Source: CAD feature listing. Evaluate the final solid. Frame: model axes, mm. A direction names the side the tool comes from. Coordinates: 2 decimals unless noted, no trailing zeros. Order: outer loops, then holes, each group sorted by start corner. A loop starts at its lowest first (then second) coordinate and runs counter-clockwise, first axis right, second up. Notation, with made-up numbers: (28.5, -33) -> (42.5, -33) arc R24 cw to (42.5, -8) -> close; hole circle Ø4 at (85, 0). An arc over 180 degrees is marked (long way). Write item = value, one per line. Start each with the question number.
Item 1: Section query A-A (y = -108.25). Output: boundary loops of the cut face in (x, z).
Item 2: Set-up query: faces 1 (the flat face through (-10, 1, 2)), 2 (the flat face through (-10, 102, 6)), 3 (the flat face through (0.1, 104.6, 4)), 4 (the flat face through (3, -111, 8)), 5 (the flat face through (42, -62.5, 2)). Return all of +Z, -Z, +X, -X, +Y, -Y with unobstructed straight access to the full face (end or side cutting, diameter ignored); none if empty.
Item 3: Mould query, pull axis X, two halves, no side actions, for faces 6 (the flat face through (0, -101, 8.5)), 7 (the flat face through (-10, -101, 6)), 8 (the cylindrical face through (40.434, -40.958, 2.281)). Classes: released by +X, released by -X, zero draft, split by the parting line, or undercut.
Item 4: Section query C-C (x = 0). Count the separate pieces of the cut face and the enclosed holes in it, then the cut area to 3 significant figures.
Item 5: Section query B-B (y = 77.5). Output: boundary loops of the cut face in (x, z) (3 decimals).
Item 6: Ray query, line 1 along Y through (x, z) = (0, 6) (3 decimals); line 2 along Y through (x, z) = (68.5, 4); line 3 along Y through (x, z) = (-14, 2.5). Return the intervals inside material, ascending. Write a range as [from, to].
Item 7: Contact query for flat-ended pins moving along their axis: pin 1 (4 mm diameter, centred on x = 14, z = 4, fed in from -Y); pin 2 (4.5 mm diameter, centred on x = 14.375, y = -77.5, fed in from -Z); pin 3 (3.5 mm diameter, centred on x = -2, y = -107.5, fed in from +Z); pin 4 (17.5 mm diameter, centred on x = -4, y = -111, fed in from -Z). Output: stop coordinate, or through.
```python
from build123d import *
from OCP.BRepFilletAPI import BRepFilletAPI_MakeFillet

# Parameters (mm, degrees)
SKETCH_1_W                   = 20
SKETCH_1_H                   = 232
EXTRUDE_1_DEPTH              = 4.5
FILLET_4_R                   = 5
EXTRUDE_START                = 4
EXTRUDE_4_DEPTH              = 4
SKETCH_9_W                   = 319.021375536
SKETCH_9_H                   = 251.112704656
SKETCH_9_W_2                 = 165.944204682
SKETCH_9_H_2                 = 200
CUT_EXTRUDE_1_DEPTH          = 4
FILLET_5_R                   = 4
HOLE_WIZARD_M6_2_D           = 6.6
HOLE_WIZARD_M6_2_CBORE_D     = 12
HOLE_WIZARD_M6_2_CBORE_DEPTH = 0.5
SKETCH_12_W                  = 65
SKETCH_12_H                  = 125
SKETCH_12_R                  = 6.25
EXTRUDE_5_DEPTH              = 4.5
SKETCH_14_R                  = 22.5
EXTRUDE_6_DEPTH              = 4.5
FILLET_6_R1                  = 10
FILLET_6_R2                  = 22.5
SKETCH_13_R                  = 6.25
CUT_EXTRUDE_2_DEPTH          = 139.39526726
HOLE_WIZARD_M6_1_D           = 5
SKETCH_17_W                  = 35
SKETCH_17_H                  = 40
CUT_EXTRUDE_3_DEPTH          = 139.395267266
FILLET_8_R                   = 5


with BuildPart() as part:
    # 草图1 → 凸台-拉伸1 (new body)
    with BuildSketch(Plane.XY):
        Rectangle(SKETCH_1_W, SKETCH_1_H)
    extrude(amount=EXTRUDE_1_DEPTH)

    # 圆角4
    fillet_4_edges = [part.edges().sort_by_distance(p)[0] for p in [
        (10, -116, 2.25),
        (-10, -116, 2.25),
        (-10, 116, 2.25),
        (10, 116, 2.25),
    ]]
    fillet(fillet_4_edges, radius=FILLET_4_R)

    # 草图8 → 凸台-拉伸4 (add)
    with BuildSketch(Plane.XY.offset(4.5).offset(EXTRUDE_START)):
        with BuildLine():
            Line((10, -91), (-10, -91))
            Line((-10, -91), (-10, -111))
            ThreePointArc((-10, -111), (-8.535533906, -114.535533906), (-5, -116))
            Line((-5, -116), (5, -116))
            ThreePointArc((5, -116), (8.535533906, -114.535533906), (10, -111))
            Line((10, -111), (10, -91))
        make_face()
        with BuildLine():
            Line((-10, 111), (-10, 91))
            Line((-10, 91), (10, 91))
            Line((10, 91), (10, 111))
            ThreePointArc((10, 111), (8.535533906, 114.535533906), (5, 116))
            Line((5, 116), (-5, 116))
            ThreePointArc((-5, 116), (-8.535533906, 114.535533906), (-10, 111))
        make_face()
    extrude(amount=-EXTRUDE_4_DEPTH)

    # 草图9 → 切除-拉伸1 (cut)
    with BuildSketch(Plane(origin=(0, 0, 0), x_dir=(-1, 0, 0), z_dir=(0, 0, -1))):
        Rectangle(SKETCH_9_W, SKETCH_9_H)
        Rectangle(SKETCH_9_W_2, SKETCH_9_H_2, mode=Mode.SUBTRACT)
    extrude(amount=-CUT_EXTRUDE_1_DEPTH, mode=Mode.SUBTRACT)

    # 圆角5
    fillet_5_edges = [part.edges().sort_by_distance(p)[0] for p in [
        (0, -91, 4.5),
        (0, 91, 4.5),
    ]]
    fillet(fillet_5_edges, radius=FILLET_5_R - 0.0001)  # a hair under: the kernel refuses the full size

    # M6 六角头螺栓的柱形沉头孔2 (through all)
    with Locations(Plane.XY.offset(8.5)):
        with Locations((0, 108.25), (0, -108.25)):
            CounterBoreHole(HOLE_WIZARD_M6_2_D / 2, HOLE_WIZARD_M6_2_CBORE_D / 2, HOLE_WIZARD_M6_2_CBORE_DEPTH)

    # 草图12 → 凸台-拉伸5 (add)
    with BuildSketch(Plane(origin=(0, 0, 0), x_dir=(-1, 0, 0), z_dir=(0, 0, -1))):
        with Locations((-42.5, 0)):
            Rectangle(SKETCH_12_W, SKETCH_12_H)
        with Locations((-52.5, 40)):
            Circle(SKETCH_12_R, mode=Mode.SUBTRACT)
        with Locations((-52.5, -40)):
            Circle(SKETCH_12_R, mode=Mode.SUBTRACT)
    extrude(amount=-EXTRUDE_5_DEPTH)

    # 草图14 → 凸台-拉伸6 (add)
    with BuildSketch(Plane(origin=(0, 0, 0), x_dir=(-1, 0, 0), z_dir=(0, 0, -1))):
        with Locations((0, 77.5)):
            Circle(SKETCH_14_R)
        with Locations((0, -77.5)):
            Circle(SKETCH_14_R)
    extrude(amount=-EXTRUDE_6_DEPTH)

    # 圆角6: one fillet with a radius per group of edges: ONE call of the kernel's fillet builder (fillet() takes one radius for all edges)
    fillet_6_edges_1 = [part.edges().sort_by_distance(p)[0] for p in [
        (16.770509831, 62.5, 2.25),
        (-10, 57.344355629, 2.25),
        (16.770509831, -62.5, 2.25),
        (-10, -57.344355629, 2.25),
    ]]
    fillet_6_edges_2 = [part.edges().sort_by_distance(p)[0] for p in [
        (75, 62.5, 2.25),
        (75, -62.5, 2.25),
    ]]
    fillet_6 = BRepFilletAPI_MakeFillet(part.part.solid().wrapped)
    for e in fillet_6_edges_1:
        fillet_6.Add(FILLET_6_R1, e.wrapped)
    for e in fillet_6_edges_2:
        fillet_6.Add(FILLET_6_R2, e.wrapped)
    add(Compound.cast(fillet_6.Shape()), mode=Mode.REPLACE)

    # 草图13 → 切除-拉伸2 (cut, through all)
    with BuildSketch(Plane(origin=(0, 0, 0), x_dir=(-1, 0, 0), z_dir=(0, 0, -1))):
        with Locations((0, 77.5)):
            Circle(SKETCH_13_R)
        with Locations((0, -77.5)):
            Circle(SKETCH_13_R)
    extrude(amount=-CUT_EXTRUDE_2_DEPTH, mode=Mode.SUBTRACT)

    # M6 螺纹孔1 (through all)
    with Locations(Plane(origin=(0, 0, 0), x_dir=(-1, 0, 0), z_dir=(0, 0, -1))):
        with Locations((-66.875, 40), (-52.5, 54.375), (-38.125, 40), (-52.5, 25.625), (-52.5, -25.625), (-38.125, -40), (-66.875, -40), (-52.5, -54.375), (0, -63.125), (14.375, -77.5), (-14.375, -77.5), (0, -91.875), (0, 91.875), (14.375, 77.5), (-14.375, 77.5), (0, 63.125)):
            Hole(HOLE_WIZARD_M6_1_D / 2)

    # 草图17 → 切除-拉伸3 (cut, through all)
    with BuildSketch(Plane(origin=(0, 0, 0), x_dir=(-1, 0, 0), z_dir=(0, 0, -1))):
        with Locations((-22.5, 0)):
            Rectangle(SKETCH_17_W, SKETCH_17_H)
    extrude(amount=-CUT_EXTRUDE_3_DEPTH, mode=Mode.SUBTRACT)

    # 圆角8
    fillet_8_edges = [part.edges().sort_by_distance(p)[0] for p in [
        (40, -20, 2.25),
        (40, 20, 2.25),
        (5, 20, 2.25),
        (5, -20, 2.25),
    ]]
    fillet(fillet_8_edges, radius=FILLET_8_R)


solid = part.part
```
Computed:
q1.outline = (-10, 4) -> (-3.3, 4) -> (-3.3, 8) -> (-6, 8) -> (-6, 8.5) -> (-10, 8.5) -> close; (3.3, 4) -> (10, 4) -> (10, 8.5) -> (6, 8.5) -> (6, 8) -> (3.3, 8) -> close
q2.face_1 = +Z, -Z, -X
q2.face_2 = +Z, -X, +Y
q2.face_3 = -Z, +X, -X, +Y
q2.face_4 = +Z
q2.face_5 = +Z, -Z, +X, -Y
q3.face_6 = zero draft
q3.face_7 = released by -X
q3.face_8 = undercut
q4.separate_pieces = 9
q4.enclosed_holes = 0
q4.area = 823 mm^2
q5.outline = (-22.5, 0) -> (-16.875, 0) -> (-16.875, 4.5) -> (-22.5, 4.5) -> close; (-11.875, 0) -> (-6.25, 0) -> (-6.25, 4.5) -> (-11.875, 4.5) -> close; (6.25, 0) -> (11.875, 0) -> (11.875, 4.5) -> (6.25, 4.5) -> close; (16.875, 0) -> (22.5, 0) -> (22.5, 4.5) -> (16.875, 4.5) -> close
q6.line_1 = [-116, -111.55], [-104.95, -94.375], [94.375, 104.95], [111.55, 116]
q6.line_2 = [-55.82, -41.9], [-38.1, 38.1], [41.9, 55.82]
q6.line_3 = [-95.11, -79.97], [-75.03, -59.89], [59.89, 75.03], [79.97, 95.11]
q7.pin_1 = -96.53
q7.pin_2 = through
q7.pin_3 = 8
q7.pin_4 = 4
